from build123d import *

# Parameters (mm, degrees)
BOSS_EXTRUDE1_DEPTH     = 5
SKETCH2_R               = 15
SKETCH2_R_2             = 12
SKETCH2_R_3             = 2
CUT_EXTRUDE1_DEPTH      = 6
CUT_EXTRUDE1_DEPTH_BACK = 6


with BuildPart() as part:
    # Sketch1 → Boss-Extrude1 (new body, symmetric)
    with BuildSketch(Plane.XY):
        Polygon((-184.95, 0), (184.95, 0), (184.95, 158), (14.95, 158), (10.05, 169), (-184.95, 169), align=None)
    extrude(amount=BOSS_EXTRUDE1_DEPTH, both=True)

    # Sketch2 → Cut-Extrude1 (cut, two sides)
    with BuildSketch(Plane.XY) as cut_extrude1_sk:
        with Locations((23.05, 71)):
            Circle(SKETCH2_R)
        with Locations((55.55, 83.2)):
            Circle(SKETCH2_R)
        with Locations((89.75, 78.4)):
            Circle(SKETCH2_R)
        with Locations((122.25, 64)):
            Circle(SKETCH2_R)
        with Locations((26.55, 109.2)):
            Circle(SKETCH2_R)
        with Locations((59.05, 121.4)):
            Circle(SKETCH2_R)
        with Locations((93.25, 116.6)):
            Circle(SKETCH2_R)
        with Locations((125.75, 102.2)):
            Circle(SKETCH2_R)
        with Locations((-14.95, 59)):
            Circle(SKETCH2_R)
        with Locations((-28.55, 114)):
            Circle(SKETCH2_R_2)
        with Locations((-55.05, 128)):
            Circle(SKETCH2_R_2)
        with Locations((-84.55, 127.3)):
            Circle(SKETCH2_R_2)
        with Locations((-7.65, 163)):
            Circle(SKETCH2_R_3)
        with Locations((-169.45, 163)):
            Circle(SKETCH2_R_3)
        with Locations((-173.95, 15.5)):
            Circle(SKETCH2_R_3)
        with Locations((0.75, 11.5)):
            Circle(SKETCH2_R_3)
        with Locations((173.45, 15.5)):
            Circle(SKETCH2_R_3)
        with Locations((177.75, 151.5)):
            Circle(SKETCH2_R_3)
    extrude(amount=CUT_EXTRUDE1_DEPTH, mode=Mode.SUBTRACT)
    extrude(cut_extrude1_sk.sketch, amount=-CUT_EXTRUDE1_DEPTH_BACK, mode=Mode.SUBTRACT)


solid = part.part
Here's how the part is built. I have some questions about the finished solid (model axes, mm). A direction names the side the tool comes from. Round coordinates to 2 decimals unless told otherwise and drop trailing zeros. Order: outer loops, then holes, each group sorted by start corner. A loop starts at its lowest first (then second) coordinate and runs counter-clockwise, first axis right, second up. Notation, with made-up numbers: M 47,4.5 L 51,4.5 A22 ccw 51,14.5 Z; hole C 54.5,88 d6. An arc over 180 degrees is marked long. Return JSON: item names as keys, results as strings. Group by question number.
1. If we mould it in two halves opening along Y, with no side actions, what happens to faces 1 (the face through (-86, 169, 0)), 2 (the face through (-3, 86, 5)), 3 (the face through (118.998, 49.357, 0.07)), 4 (the face through (-3, 0, 0))? For each: pulls with the +Y half, pulls with the -Y half, needs draft (parallel to the pull), parting line crosses it, or undercut.
2. On a 3-axis mill with a long thin cutter (end or side, diameter ignored), from which of +Z, -Z, +X, -X, +Y, -Y can I reach the whole of each face in a straight line? I mean faces 5 (the face through (101, 158, 0)), 6 (the face through (-31.151, 102.285, 0.07)). Say none if no direction works.
3. If we section it at C-C on x = 89: List the corners of the cut face in (y, z) for me, then the cut area to 3 significant figures.
4. Please list where these lines run through material, in increasing order: probe 1 along X at (y, z) = (95.5, 2.5); probe 2 along Y at (x, z) = (-169.45, 1.25); probe 3 along Y at (x, z) = (59.05, 1.5).
5. If we section it at B-B on z = -0.5: State how many separate pieces and enclosed holes the cut face has, then the cut area to 3 significant figures.
6. If we section it at A-A on x = -55.05: List the corners of the cut face in (y, z) for me, then the cut area to 3 significant figures.
7. I'm going to push flat-ended pins straight in: pin 1 Ø24 at (x, y) = (89.75, 78.4) entering from -Z; pin 2 Ø3 at (x, z) = (139.5, -1) entering from +Y. Where does each tip first touch, or does it pass through?
Reply:
{
 "1": {"face 1": "pulls with the +Y half", "face 2": "needs draft", "face 3": "undercut", "face 4": "pulls with the -Y half"},
 "2": {"face 5": "+Z, -Z, +X, +Y", "face 6": "+Z, -Z"},
 "3": {"outline": "M 0,-5 L 63.42,-5 L 63.42,5 L 0,5 Z; M 93.38,-5 L 102.21,-5 L 102.21,5 L 93.38,5 Z; M 130.99,-5 L 158,-5 L 158,5 L 130.99,5 Z", "area": "993 mm^2"},
 "4": {"probe 1": "-184.95 to 20.44, 32.66 to 46.96, 64.14 to 112.33, 139.17 to 184.95", "probe 2": "0 to 161, 165 to 169", "probe 3": "0 to 68.61, 97.79 to 106.4, 136.4 to 158"},
 "5": {"separate pieces": "1", "enclosed holes": "18", "area": "52,800 mm^2"},
 "6": {"outline": "M 0,-5 L 116,-5 L 116,5 L 0,5 Z; M 140,-5 L 169,-5 L 169,5 L 140,5 Z", "area": "1,450 mm^2"},
 "7": {"pin 1": "through", "pin 2": "y = 158"}
}
